from build123d import *

# Parameters (mm, degrees)
SKETCH1_R                     = 1.5
BOSS_EXTRUDE1_DEPTH           = 3
SKETCH4_W                     = 3.5
SKETCH4_H                     = 12
BOSS_EXTRUDE3_DEPTH           = 10.5
SKETCH5_W                     = 2
SKETCH5_H                     = 12
BOSS_EXTRUDE4_DEPTH           = 1.1
SKETCH6_W                     = 0.2
SKETCH6_H                     = 3
BOSS_EXTRUDE5_DEPTH           = 0.5
CHAMFER1_SIZE                 = 10.5
SKETCH10_R                    = 1.5
BOSS_EXTRUDE6_DEPTH           = 2
CSK_FOR_M4_SFHCS1_D           = 4
CSK_FOR_M4_SFHCS1_DEPTH       = 30.798278762
CSK_FOR_M4_SFHCS1_CSINK_D     = 7.5
CSK_FOR_M4_SFHCS1_CSINK_ANGLE = 90
CSK_FOR_M4_SFHCS1_TIP         = 1.201721238


with BuildPart() as part:
    # Sketch1 → Boss-Extrude1 (new body)
    with BuildSketch(Plane(origin=(0, 0, 0), x_dir=(1, 0, 0), z_dir=(0, 1, 0))):
        with BuildLine():
            Line((-49, 6), (49, 6))
            ThreePointArc((49, 6), (55, 0), (49, -6))
            Line((49, -6), (-49, -6))
            ThreePointArc((-49, -6), (-55, 0), (-49, 6))
        make_face()
        with Locations(Location((-51.5, 0, 0), (0, 0, 270))):
            Circle(SKETCH1_R, mode=Mode.SUBTRACT)
        with Locations(Location((51.5, 0, 0), (0, 0, 270))):
            Circle(SKETCH1_R, mode=Mode.SUBTRACT)
    extrude(amount=BOSS_EXTRUDE1_DEPTH)

    # Sketch4 → Boss-Extrude3 (add)
    with BuildSketch(Plane.XZ):
        with Locations((-21.690023983, 0)):
            Rectangle(SKETCH4_W, SKETCH4_H)
        with Locations((21.690023983, 0)):
            Rectangle(SKETCH4_W, SKETCH4_H)
    extrude(amount=BOSS_EXTRUDE3_DEPTH)

    # Sketch5 → Boss-Extrude4 (add)
    with BuildSketch(Plane.XZ):
        with Locations((5, 0)):
            Rectangle(SKETCH5_W, SKETCH5_H)
        Rectangle(SKETCH5_W, SKETCH5_H)
        with Locations((10, 0)):
            Rectangle(SKETCH5_W, SKETCH5_H)
        with Locations((-5, 0)):
            Rectangle(SKETCH5_W, SKETCH5_H)
        with Locations((-10, 0)):
            Rectangle(SKETCH5_W, SKETCH5_H)
    extrude(amount=BOSS_EXTRUDE4_DEPTH)

    # Sketch6 → Boss-Extrude5 (add)
    with BuildSketch(Plane.XY.offset(6)):
        with Locations((48.9, 1.5)):
            Rectangle(SKETCH6_W, SKETCH6_H)
        with Locations((-48.9, 1.5)):
            Rectangle(SKETCH6_W, SKETCH6_H)
    extrude(amount=BOSS_EXTRUDE5_DEPTH)

    # Chamfer1
    chamfer1_edges = [part.edges().sort_by_distance(p)[0] for p in [
        (-23.440023983, 0, 0),
        (23.440023983, 0, 0),
    ]]
    chamfer(chamfer1_edges, length=CHAMFER1_SIZE - 0.0001)  # a hair under: the kernel refuses the full size

    # Sketch10 → Boss-Extrude6 (add)
    with BuildSketch(Plane(origin=(0, 3, 0), x_dir=(1, 0, 0), z_dir=(0, 1, 0))):
        with BuildLine():
            Line((-49, -6), (-49, -6.5))
            Line((-49, -6.5), (-48.8, -6.5))
            Line((-48.8, -6.5), (-48.8, -6))
            Line((-48.8, -6), (48.8, -6))
            Line((48.8, -6), (48.8, -6.5))
            Line((48.8, -6.5), (49, -6.5))
            Line((49, -6.5), (49, -6))
            ThreePointArc((49, -6), (55, 0), (49, 6))
            Line((49, 6), (-49, 6))
            ThreePointArc((-49, 6), (-55, 0), (-49, -6))
        make_face()
        with Locations(Location((-51.5, 0, 0), (0, 0, 270))):
            Circle(SKETCH10_R, mode=Mode.SUBTRACT)
        with Locations(Location((51.5, 0, 0), (0, 0, 270))):
            Circle(SKETCH10_R, mode=Mode.SUBTRACT)
    extrude(amount=BOSS_EXTRUDE6_DEPTH)

    # CSK for M4 SFHCS1
    with Locations(Plane(origin=(0, 5, 0), x_dir=(1, 0, 0), z_dir=(0, 1, 0))):
        with Locations((51.5, 0), (-51.5, 0)):
            CounterSinkHole(CSK_FOR_M4_SFHCS1_D / 2, CSK_FOR_M4_SFHCS1_CSINK_D / 2, depth=CSK_FOR_M4_SFHCS1_DEPTH, counter_sink_angle=CSK_FOR_M4_SFHCS1_CSINK_ANGLE)
            with Locations((0, 0, -(CSK_FOR_M4_SFHCS1_DEPTH + CSK_FOR_M4_SFHCS1_TIP / 2))):  # 118° drill point
                Cone(0, CSK_FOR_M4_SFHCS1_D / 2, CSK_FOR_M4_SFHCS1_TIP, mode=Mode.SUBTRACT)


solid = part.part
The model under review builds one solid part; all positions refer to its coordinate system, in mm. A direction names the side the tool comes from. Give positions to 0.01 mm unless a question says otherwise; leave off trailing zeros. Loops run counter-clockwise (first coordinate to the right, second up) from the corner with the lowest first, then second, coordinate; pieces in that order, holes last. Notation, with made-up numbers: (58, 34.5) -> (113, 34.5) arc R17 ccw to (113, 57.5) -> close; hole circle Ø8 at (-8.5, 29). An arc over 180 degrees is marked (long way). Answer as a JSON object with one key per item and string values. Group by question number.
Q1. Take a section at D-D (x = 36). Write out the cut boundary in (y, z), plus the area to 3 significant figures.
Q2. Take a section at B-B (z = 0). State how many separate pieces and enclosed holes the cut face has, plus the area to 3 significant figures.
Q3. Take a section at A-A (y = -5.5). Write out the cut boundary in (x, z), plus the area to 3 significant figures.
Q4. Wall thickness on line 1 along X through (y, z) = (4.25, 2.5); line 2 along Y through (x, z) = (-8, -4.25); line 3 along Z through (x, y) = (-51.5, 1.4): over which ranges is each line inside the solid? List them lowest first.
Q5. Tool access review of faces 1 (the flat face through (-28.76, -5.18, -0.08)), 2 (the flat face through (-1, 1, 6)), 3 (the flat face through (-19.94, -5, 0)): name each direction out of +Z, -Z, +X, -X, +Y, -Y from which nothing blocks a thin tool from reaching the whole face with its end or side.
Q6. Insertion check: pin 1 (5 mm diameter, centred on y = -6.5, z = 0.5, fed in from -X); pin 2 (0.6 mm diameter, centred on y = 1.5, z = 6.5, fed in from +X); pin 3 (0.9 mm diameter, centred on y = -0.5, z = -0.5, fed in from -X). Each pin has a flat end and moves straight along its axis. Give the tip position at first contact, or say it passes through.
Q7. Take a section at C-C (x = -51.5). Write out the cut boundary in (y, z), plus the area to 3 significant figures.
Answer below:
{
 "1": {"outline": "(0, -6) -> (5, -6) -> (5, 6) -> (0, 6) -> close", "area": "60.0 mm2"},
 "2": {"separate pieces": "3", "enclosed holes": "0", "area": "699 mm2"},
 "3": {"outline": "(-28.44, -6) -> (-19.94, -6) -> (-19.94, 6) -> (-28.44, 6) -> close; (19.94, -6) -> (28.44, -6) -> (28.44, 6) -> (19.94, 6) -> close", "area": "204 mm2"},
 "4": {"line 1": "x = -54.45 to -53.16, -49.84 to 49.84, 53.16 to 54.45", "line 2": "y = 0 to 5", "line 3": "z = -5.45 to -2, 2 to 5.45"},
 "5": {"face 1": "+Z, -Z, -X, -Y", "face 2": "+Z, +Y, -Y", "face 3": "+Z, -Z, -Y"},
 "6": {"pin 1": "stops at x = -29.94", "pin 2": "stops at x = 49", "pin 3": "stops at x = -33.89"},
 "7": {"outline": "(0, -5.45) -> (5, -5.45) -> (5, -3.75) -> (3.25, -2) -> (0, -2) -> close; (0, 2) -> (3.25, 2) -> (5, 3.75) -> (5, 5.45) -> (0, 5.45) -> close", "area": "31.5 mm2"}
}
